```python
from build123d import *

# Parameters (mm, degrees)
SKETCH1_R           = 11.1125
BOSS_EXTRUDE1_DEPTH = 19.05
SKETCH2_R           = 15.875
BOSS_EXTRUDE2_DEPTH = 12.7
CUT_EXTRUDE1_START  = -8.89
SKETCH3_R           = 15.875
CUT_EXTRUDE1_DEPTH  = 8.89
CHAMFER1_SIZE       = 1.27
CUT_EXTRUDE2_REACH  = 40.886
SKETCH4_R           = 1


with BuildPart() as part:
    # Sketch1 → Boss-Extrude1 (new body)
    with BuildSketch(Plane.XY):
        with Locations(Location((0, 0, 0), (0, 0, 180))):
            Circle(SKETCH1_R)
    extrude(amount=BOSS_EXTRUDE1_DEPTH)

    # Sketch2 → Boss-Extrude2 (add)
    with BuildSketch(Plane.XY.offset(19.05)):
        Circle(SKETCH2_R)
    extrude(amount=BOSS_EXTRUDE2_DEPTH)

    # Sketch3 → Cut-Extrude1 (cut)
    with BuildSketch(Plane.XY.offset(31.75).offset(CUT_EXTRUDE1_START)):
        Circle(SKETCH3_R)
        Polygon((12.831609733, 0), (6.415804866, 11.1125), (-6.415804866, 11.1125), (-12.831609733, 0), (-6.415804866, -11.1125), (6.415804866, -11.1125), align=None, mode=Mode.SUBTRACT)
    extrude(amount=CUT_EXTRUDE1_DEPTH, mode=Mode.SUBTRACT)

    # Chamfer1
    chamfer1_edges = [part.edges().sort_by_distance(p)[0] for p in [
        (-15.875, 0, 22.86),
    ]]
    chamfer(chamfer1_edges, length=CHAMFER1_SIZE)

    # Cut-Loft1: read off the stored shape, not the designer's step
    # Cut-Loft1: loft between two sections, ruled curve by curve
    cut_loft1_from = [
        Edge.make_bspline([(2.35183174, 9.256296648, 0), (-16.160761555, 13.959960127, 0), (-20.864425035, -4.552633168, 0), (-2.35183174, -9.256296648, 0), (16.160761555, -13.959960127, 0), (20.864425035, 4.552633168, 0), (2.35183174, 9.256296648, 0)], [0, 0, 0, 0, 0.5, 0.5, 0.5, 1, 1, 1, 1], 3, [1, 0.333333333, 0.333333333, 1, 0.333333333, 0.333333333, 1]),
    ]
    cut_loft1_to = [
        Edge.make_bspline([(2.644109425, 4.759906548, 22.86), (-6.875703672, 10.048125398, 22.86), (-12.163922522, 0.528312301, 22.86), (-2.644109425, -4.759906548, 22.86), (6.875703672, -10.048125398, 22.86), (12.163922522, -0.528312301, 22.86), (2.644109425, 4.759906548, 22.86)], [0, 0, 0, 0, 0.5, 0.5, 0.5, 1, 1, 1, 1], 3, [1, 0.333333333, 0.333333333, 1, 0.333333333, 0.333333333, 1]),
    ]
    cut_loft1 = Solid(Shell([*[Face.make_surface_from_curves(cut_loft1_from[k], cut_loft1_to[k]) for k in range(1)], Face(Wire(cut_loft1_from)), Face(Wire(cut_loft1_to))]))
    add(cut_loft1, mode=Mode.SUBTRACT)

    # Sketch4 → Cut-Extrude2 (cut, up to next)
    with BuildSketch(Plane.XY.offset(31.75), mode=Mode.PRIVATE) as cut_extrude2_sk1:
        with Locations((0, 4.445)):
            Circle(SKETCH4_R)
    cut_extrude2_tool1 = extrude(cut_extrude2_sk1.sketch, amount=-CUT_EXTRUDE2_REACH, mode=Mode.PRIVATE) & part.part
    # Sketch4 → Cut-Extrude2 (cut, up to next)
    with BuildSketch(Plane.XY.offset(31.75), mode=Mode.PRIVATE) as cut_extrude2_sk2:
        with Locations((3.84948292, -2.2225)):
            Circle(SKETCH4_R)
    cut_extrude2_tool2 = extrude(cut_extrude2_sk2.sketch, amount=-CUT_EXTRUDE2_REACH, mode=Mode.PRIVATE) & part.part
    # Sketch4 → Cut-Extrude2 (cut, up to next)
    with BuildSketch(Plane.XY.offset(31.75), mode=Mode.PRIVATE) as cut_extrude2_sk3:
        with Locations((-3.84948292, -2.2225)):
            Circle(SKETCH4_R)
    cut_extrude2_tool3 = extrude(cut_extrude2_sk3.sketch, amount=-CUT_EXTRUDE2_REACH, mode=Mode.PRIVATE) & part.part
    add(cut_extrude2_tool1.solids().sort_by_distance((0, 4.445, 31.75))[0], mode=Mode.SUBTRACT)
    add(cut_extrude2_tool2.solids().sort_by_distance((3.849483, -2.2225, 31.75))[0], mode=Mode.SUBTRACT)
    add(cut_extrude2_tool3.solids().sort_by_distance((-3.849483, -2.2225, 31.75))[0], mode=Mode.SUBTRACT)


solid = part.part
```
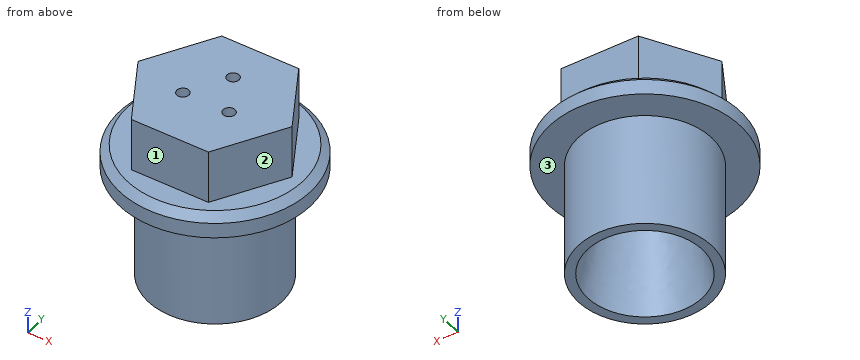
Input: part model. Units: mm. Frame: model coordinates. Face numbers are marked on the shaded views. A direction names the side the tool comes from. Give positions to 0.01 mm unless a question says otherwise; leave off trailing zeros. Return JSON: item names as keys, results as strings.
Item 1: Ray query, probe 1 along Y at (x, z) = (0, 25) (1 decimal); probe 2 along Y at (x, z) = (-3, 13.5); probe 3 along Z at (x, y) = (2.5, 0.5). Return the intervals inside material, ascending.
Solutions:
{"probe 1": "-11.1 to 3.4, 5.4 to 11.1", "probe 2": "-10.7 to -6.4, 6.4 to 10.7", "probe 3": "22.86 to 31.75"}
Item 2: Access query for the marked faces 1, 2 and 3. Directions: +Z, -Z, +X, -X, +Y, -Y. A direction counts if a zero-diameter tool reaches every point of the face in a straight line with its end or side. Return the directions, or none.
Solutions:
{"face 1": "+Z, +X, -X, -Y", "face 2": "+Z, +X, -Y", "face 3": "-Z"}
Item 3: First-contact query: P1, Ø3.5, axis at x = 0, y = 0, coming from the -Z side; P2, Ø4.5, axis at x = 3, z = 25.5, coming from the -Y side; P3, Ø1.5, axis at y = 2.5, z = 27, coming from the -X side. Flat tips, straight axial feed; report the tip coordinate or a pass-through.
Solutions:
{"P1": "z = 22.86", "P2": "y = -11.11", "P3": "x = -11.82"}
